Verification items for the finished model (mm, model axes). A direction names the side the tool comes from. Give positions to 0.01 mm unless a question says otherwise; leave off trailing zeros. Order: outer loops, then holes, each group sorted by start corner. A loop starts at its lowest first (then second) coordinate and runs counter-clockwise, first axis right, second up. Notation, with made-up numbers: (72.25, 39.25) - (114.25, 39.25) arc R20 ccw to (114.25, 51.25) - close; hole circle Ø3 at (-15.75, 29.25). An arc over 180 degrees is marked (long way). Answer as a JSON object with one key per item and string values.
```python
from build123d import *

# Parameters (mm, degrees)
BOSS_EXTRUDE1_DEPTH = 26.5
BOSS_EXTRUDE2_START = 3
BOSS_EXTRUDE2_DEPTH = 3
BOSS_EXTRUDE3_DEPTH = 3


with BuildPart() as part:
    # Sketch1 → Boss-Extrude1 (new body)
    with BuildSketch(Plane(origin=(0, 0, 0), x_dir=(1, 0, 0), z_dir=(0, 1, 0))):
        with BuildLine():
            Line((29.08394086, 70.214844471), (27.935890563, 67.443205873))
            ThreePointArc((27.935890563, 67.443205873), (0, 73), (-27.935890563, 67.443205873))
            Line((-27.935890563, 67.443205873), (-29.08394086, 70.214844471))
            ThreePointArc((-29.08394086, 70.214844471), (0, 76), (29.08394086, 70.214844471))
        make_face()
    extrude(amount=BOSS_EXTRUDE1_DEPTH)

    # Sketch2 → Boss-Extrude2 (add)
    with BuildSketch(Plane.XZ.offset(BOSS_EXTRUDE2_START)):
        with BuildLine():
            Line((27.935890563, -67.443205873), (29.08394086, -70.214844471))
            ThreePointArc((29.08394086, -70.214844471), (0, -76), (-29.08394086, -70.214844471))
            Line((-29.08394086, -70.214844471), (-27.935890563, -67.443205873))
            ThreePointArc((-27.935890563, -67.443205873), (0, -73), (27.935890563, -67.443205873))
        make_face()
    extrude(amount=-BOSS_EXTRUDE2_DEPTH)

    # Sketch3 → Boss-Extrude3 (add)
    with BuildSketch(Plane.XZ.offset(3)):
        with BuildLine():
            Line((27.935890563, -67.443205873), (28.509915711, -68.829025172))
            ThreePointArc((28.509915711, -68.829025172), (0, -74.519275475), (-28.509915711, -68.829025172))
            Line((-28.509915711, -68.829025172), (-27.935890563, -67.443205873))
            ThreePointArc((-27.935890563, -67.443205873), (0, -73.019276769), (27.935890563, -67.443205873))
        make_face()
    extrude(amount=BOSS_EXTRUDE3_DEPTH)


solid = part.part
```
(1) Section check C-C (y = 13.5). Record the cut outline in (x, z), then the cut area to 3 significant figures.
Computed values:
{"outline": "(-29.08, -70.21) arc R76 ccw to (29.08, -70.21) - (27.94, -67.44) arc R73 cw to (-27.94, -67.44) - close", "area": "176 mm²"}
(2) Access from +Z, -Z, +X, -X, +Y, -Y to the whole of each face (thin tool, end or side, straight path). Record for faces 1 (the cylindrical face through (0.41, -4.48, -74.52)), 2 (the cylindrical face through (0, 12, -73)).
Computed values:
{"face 1": "-Z, -Y", "face 2": "+Z, +Y, -Y"}
(3) Gauge pin test, flat ends, axial feed: pin 1 Ø1.5 at (x, y) = (-12.5, 18) entering from +Z; pin 2 Ø3.5 at (x, z) = (-12, -71) entering from -Y; pin 3 Ø1 at (x, y) = (-3.5, 21) entering from -Z; pin 4 Ø1.5 at (x, z) = (-14, -74.5) entering from -Y. Record the tip position at first contact, or that the pin passes through.
Computed values:
{"pin 1": "stops at z = -71.79", "pin 2": "stops at y = -6", "pin 3": "stops at z = -75.94", "pin 4": "stops at y = -3"}
(4) Material ranges on line 1 along Y through (x, z) = (-10.5, -74); line 2 along Z through (x, y) = (-24, 2); line 3 along Z through (x, y) = (-15, 23.5), recorded low to high. Write a range as [from, to].
Computed values:
{"line 1": "y = [-3, 26.5]", "line 2": "z = [-72.11, -68.94]", "line 3": "z = [-74.51, -71.44]"}
